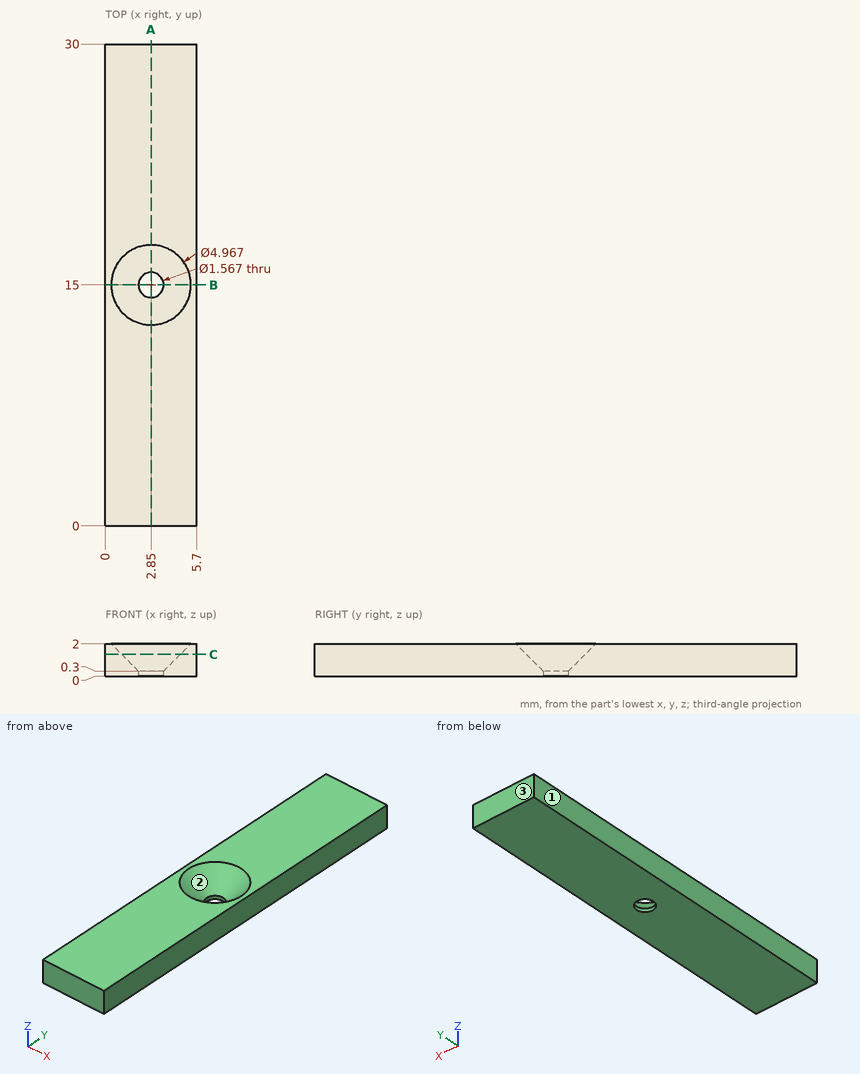
Verification items for this drawing (mm, ordinates from the low corner). Coordinates: 2 decimals unless noted, no trailing zeros. Order: outer loops, then holes, each group sorted by start corner. A loop starts at its lowest first (then second) coordinate and runs counter-clockwise, first axis right, second up. Notation, with made-up numbers: M 12,-15 L 61,-15 A22 cw 61,13 Z; hole C 54.25,-30 d1. An arc over 180 degrees is marked long. One line per item, written item: value. Start each with the question number.
Item 1: Mould release check, pull along X, two halves, no side actions. Record for the marked faces 1, 2 and 3: pulls with the +X half, pulls with the -X half, needs draft (parallel to the pull), parting line crosses it, or undercut.
Item 2: Thickness scan on probe 1 along Y at (x, z) = (4.05, 0.95); probe 2 along Y at (x, z) = (3.4, 1.15). Record the ranges inside material, lowest first.
Item 3: Depth check by flat-ended pin: P1, Ø2, axis at x = 2.85, y = 15, coming from the +Z side. Enter the tip coordinate at first touch or a pass-through.
Item 4: Sectioned sample at C-C on z = 1.35. Record the cut outline in (x, y), then the cut area to 3 significant figures.
Item 5: Sectioned sample at B-B on y = 15. Record the cut outline in (x, z), then the cut area to 3 significant figures.
Item 6: Sectioned sample at A-A on x = 2.85. Record the cut outline in (y, z).
Calculated:
1. face 1: pulls with the -X half
1. face 2: undercut
1. face 3: needs draft
2. probe 1: 0 to 14.22, 15.78 to 30
2. probe 2: 0 to 13.46, 16.54 to 30
3. P1: z = 0.52
4. outline: M 0,0 L 5.7,0 L 5.7,30 L 0,30 Z; hole C 2.85,15 d3.67
4. area: 160 mm^2
5. outline: M 0,0 L 2.07,0 L 2.07,0.3 L 0.37,2 L 0,2 Z; M 3.63,0 L 5.7,0 L 5.7,2 L 5.33,2 L 3.63,0.3 Z
5. area: 5.38 mm^2
6. outline: M 0,0 L 14.22,0 L 14.22,0.3 L 12.52,2 L 0,2 Z; M 15.78,0 L 30,0 L 30,2 L 17.48,2 L 15.78,0.3 Z
